Verification items for the finished model (mm, model axes). Coordinates: 2 decimals unless noted, no trailing zeros. Write each loop counter-clockwise with the first axis right and the second up, starting at its lowest first coordinate (ties: lowest second). Pieces come first, ordered by that corner, then holes. Notation, with made-up numbers: M -19,61 L 25,61 A10 cw 25,70 Z; hole C 7,71.5 d5. An arc over 180 degrees is marked long. One line per item, written item: value.
```python
from build123d import *

# Parameters (mm, degrees)
SKETCH036_W     = 92
SKETCH036_H     = 92
PAD022_DEPTH    = 4
SKETCH037_R     = 2.6
POCKET012_DEPTH = 4.001
FILLET001_R     = 5


with BuildPart() as part:
    # Sketch036 → Pad022 (new body)
    with BuildSketch(Plane.XY):
        Rectangle(SKETCH036_W, SKETCH036_H)
    extrude(amount=PAD022_DEPTH)

    # Sketch037 (on Face6 of Pad022) → Pocket012 (cut, through all)
    with BuildSketch(Plane.XY.offset(4)):
        with Locations((-39, 38)):
            Circle(SKETCH037_R)
        with Locations((-39, -38)):
            Circle(SKETCH037_R)
        with Locations((39, -38)):
            Circle(SKETCH037_R)
        with Locations((39, 38)):
            Circle(SKETCH037_R)
    extrude(amount=-POCKET012_DEPTH, mode=Mode.SUBTRACT)

    # Fillet001
    fillet001_edges = [part.edges().sort_by_distance(p)[0] for p in [
        (46, -46, 2),
        (-46, -46, 2),
        (-46, 46, 2),
        (46, 46, 2),
    ]]
    fillet(fillet001_edges, radius=FILLET001_R)


solid = part.part
```
Item 1: Scan lines: line 1 (Y direction, x = -39, z = 1); line 2 (Y direction, x = -37.5, z = 2.75). Record each from-to range of solid material in increasing order.
The answers:
line 1: y = -46 to -40.6, -35.4 to 35.4, 40.6 to 46
line 2: y = -46 to -40.12, -35.88 to 35.88, 40.12 to 46
Item 2: Cross-section at A-A, the plane y = 38. Enter the section's corners in (x, z), and give its area (3 significant figures).
The answers:
outline: M -46,0 L -41.6,0 L -41.6,4 L -46,4 Z; M -36.4,0 L 36.4,0 L 36.4,4 L -36.4,4 Z; M 41.6,0 L 46,0 L 46,4 L 41.6,4 Z
area: 326 mm²
Item 3: Go/stop test with flat-tipped pins: P1, Ø3, axis at x = 39, y = 38, coming from the -Z side; P2, Ø6, axis at x = -39, y = -38, coming from the +Z side. Record where each tip stops, or that it passes through.
The answers:
P1: passes through
P2: stops at z = 4
Item 4: Draft check along X on faces 1 (the face through (-45, 44, 2)), 2 (the face through (36.937, -39.582, 2.028)), 3 (the face through (44, -45, 2)). Enter one of: released by +X, released by -X, zero draft, split by the parting line, or undercut.
The answers:
face 1: released by -X
face 2: undercut
face 3: released by +X
Item 5: Cross-section at B-B, the plane x = 39. Enter the section's corners in (y, z).
The answers:
outline: M -46,0 L -40.6,0 L -40.6,4 L -46,4 Z; M -35.4,0 L 35.4,0 L 35.4,4 L -35.4,4 Z; M 40.6,0 L 46,0 L 46,4 L 40.6,4 Z
